Here's how the part is built. I have some questions about the finished solid (model axes, mm). A direction names the side the tool comes from. Give positions to 0.01 mm unless a question says otherwise; leave off trailing zeros. Order: outer loops, then holes, each group sorted by start corner. A loop starts at its lowest first (then second) coordinate and runs counter-clockwise, first axis right, second up. Notation, with made-up numbers: M 41,-31 L 97,-31 A28 ccw 97,5 Z; hole C 37.25,41 d4. An arc over 180 degrees is marked long. Use one line per item in the form item = value.
from build123d import *

# Parameters (mm, degrees)
BOSS_EXTRUDE1_DEPTH = 110
SKETCH2_W           = 80
SKETCH2_H           = 80
BOSS_EXTRUDE2_DEPTH = 20
SKETCH3_R           = 15
CUT_EXTRUDE1_DEPTH  = 20
BOSS_EXTRUDE3_START = 5
BOSS_EXTRUDE3_DEPTH = 5
BOSS_EXTRUDE4_DEPTH = 10
HOLE1_D             = 20
SKETCH9_R           = 5
BOSS_EXTRUDE5_DEPTH = 15
LPATTERN1_COUNT     = 2
LPATTERN1_PITCH     = 65


with BuildPart() as part:
    # Sketch1 → Boss-Extrude1 (new body)
    with BuildSketch(Plane.XY):
        Polygon((-40, 20), (-40, 0), (40, 0), (40, 20), (30, 20), (30, 10), (-30, 10), (-30, 20), align=None)
    extrude(amount=BOSS_EXTRUDE1_DEPTH)

    # Sketch2 → Boss-Extrude2 (add)
    with BuildSketch(Plane(origin=(0, 0, 0), x_dir=(-1, 0, 0), z_dir=(0, 0, -1))):
        with Locations((0, 40)):
            Rectangle(SKETCH2_W, SKETCH2_H)
    extrude(amount=-BOSS_EXTRUDE2_DEPTH)

    # Sketch3 → Cut-Extrude1 (cut)
    with BuildSketch(Plane.XY.offset(20)):
        with Locations((0, 80)):
            Circle(SKETCH3_R)
    extrude(amount=-CUT_EXTRUDE1_DEPTH, mode=Mode.SUBTRACT)

    # Sketch4 → Boss-Extrude3 (add)
    with BuildSketch(Plane.XY.offset(20).offset(BOSS_EXTRUDE3_START)):
        with BuildLine():
            Line((-20, 80), (-15, 80))
            ThreePointArc((-15, 80), (0, 65), (15, 80))
            Line((15, 80), (20, 80))
            ThreePointArc((20, 80), (0, 60), (-20, 80))
        make_face()
    extrude(amount=-BOSS_EXTRUDE3_DEPTH)

    # Sketch6 → Boss-Extrude4 (add)
    with BuildSketch(Plane(origin=(0, 10, 0), x_dir=(1, 0, 0), z_dir=(0, 1, 0))):
        with BuildLine():
            Line((-15, -110), (15, -110))
            ThreePointArc((15, -110), (0, -125), (-15, -110))
        make_face()
    extrude(amount=-BOSS_EXTRUDE4_DEPTH)

    # Hole1 (through all)
    with Locations(Plane(origin=(0, 10, 0), x_dir=(1, 0, 0), z_dir=(0, 1, 0))):
        with Locations((0, -110)):
            Hole(HOLE1_D / 2)

    # Sketch9 → Boss-Extrude5 (add)
    with BuildSketch(Plane(origin=(40, 0, 0), x_dir=(0, 0, -1), z_dir=(1, 0, 0))):
        with BuildLine():
            Line((-80, 60), (-80, 0))
            Line((-80, 0), (-60, 0))
            Line((-60, 0), (-60, 60))
            ThreePointArc((-60, 60), (-70, 70), (-80, 60))
        make_face()
        with Locations((-70, 60)):
            Circle(SKETCH9_R, mode=Mode.SUBTRACT)
    boss_extrude5 = extrude(amount=-BOSS_EXTRUDE5_DEPTH)

    # LPattern1: Boss-Extrude5 ×2
    with Locations(*[(-i * LPATTERN1_PITCH, 0, 0) for i in range(1, LPATTERN1_COUNT)]):
        add(boss_extrude5)


solid = part.part
Q1. I'm going to push flat-ended pins straight in: pin 1 Ø11 at (x, z) = (-37.5, 38) entering from +Y; pin 2 Ø3 at (x, y) = (27, 40.5) entering from +Z; pin 3 Ø6 at (x, y) = (32, 10.5) entering from +Z. Where does each tip first touch, or does it pass through?
Found:
pin_1 = 20
pin_2 = 80
pin_3 = 110
Q2. I want a section at C-C on y = 51. Write out the boundary of the cut face in (x, z).
Found:
outline = M -40,0 L 40,0 L 40,20 L -40,20 Z; M -40,60 L -25,60 L -25,80 L -40,80 Z; M 25,60 L 40,60 L 40,80 L 25,80 Z
Q3. I want a section at D-D on z = 102. Write out the boundary of the cut face in (x, y).
Found:
outline = M -40,0 L -6,0 L -6,10 L -30,10 L -30,20 L -40,20 Z; M 6,0 L 40,0 L 40,20 L 30,20 L 30,10 L 6,10 Z
Q4. On a 3-axis mill with a long thin cutter (end or side, diameter ignored), from which of +Z, -Z, +X, -X, +Y, -Y can I reach the whole of each face in a straight line? I mean faces 1 (the face through (-25, 40, 70)), 2 (the face through (-35, 20, 40)), 3 (the face through (30, 15, 40)). Say none if no direction works.
Found:
face_1 = +Z, +Y
face_2 = +X, -X, +Y
face_3 = +Y
Q5. I need wall thicknesses on L1, parallel to Z at x = 0, y = 7; L2, parallel to Z at x = -28, y = 29; L3, parallel to Z at x = -32, y = 61. Which ranges of each line are inside material? Lowest first, please.
Found:
L1 = 0 to 100, 120 to 125
L2 = 0 to 20, 60 to 80
L3 = 0 to 20, 60.05 to 65.1, 74.9 to 79.95
Q6. Thinking about a two-plate mould opening in Z: for faces 4 (the face through (0, 5, 125)), 5 (the face through (-1, 41, 0)), 6 (the face through (25, 40, 70)), 7 (the face through (33, 40, 60)), which applies, +Z half, -Z half, draft (parallel to the pull), parting line (faces both ways), or undercut?
Found:
face_4 = +Z half
face_5 = -Z half
face_6 = draft
face_7 = undercut
Q7. I want a section at B-B on z = 70. Write out the boundary of the cut face in (x, y).
Found:
outline = M -40,0 L 40,0 L 40,55 L 25,55 L 25,10 L -25,10 L -25,55 L -40,55 Z; M -40,65 L -25,65 L -25,70 L -40,70 Z; M 25,65 L 40,65 L 40,70 L 25,70 Z
Q8. I want a section at A-A on x = 0. Write out the boundary of the cut face in (y, z).
Found:
outline = M 0,0 L 65,0 L 65,25 L 60,25 L 60,20 L 10,20 L 10,100 L 0,100 Z; M 0,120 L 10,120 L 10,125 L 0,125 Z
